Autodesk Fusion 360 part; units mm, degrees
sketch "Sketch1" plane through (0, 0, 0) normal (0, 0, 1) x (1, 0, 0)
  line L0 (0, 0) -> (115, 0)
  line L1 (115, 0) -> (115, 39)
  line L2 (115, 39) -> (0, 39)
  line L3 (0, 39) -> (0, 0)
  circle A0 centre (5, 34) radius 1.6
  circle A1 centre (5, 5) radius 1.6
  circle A2 centre (110, 5) radius 1.6
  circle A3 centre (110, 34) radius 1.6
  dimension "d1" = 115
  dimension "d2" = 39
  dimension "d3" = 3.2
  dimension "d4" = 5
  dimension "d5" = 5
  dimension "d6" = 3.2
  dimension "d7" = 5
  dimension "d8" = 5
  dimension "d9" = 3.2
  dimension "d10" = 3.2
  dimension "d11" = 5
  dimension "d12" = 5
  dimension "d13" = 5
  dimension "d14" = 5
extrude "Extrude1" add sketch "Sketch1" along normal blind 2.7
fillet "Fillet1" radius 6 4 edges at (115, 39, 1.35) (115, 0, 1.35) (0, 39, 1.35) (0, 0, 1.35)
Work out the finished part from the listing and answer in its coordinate system (mm). Give positions to 0.01 mm unless a question says otherwise; leave off trailing zeros. Write each loop counter-clockwise with the first axis right and the second up, starting at its lowest first coordinate (ties: lowest second). Pieces come first, ordered by that corner, then holes.
(1) The part is cut by section B-B on x = 5. Write down the section's boundary in (y, z), plus the area to 3 significant figures.
Final values:
outline: (0.08, 0) - (3.4, 0) - (3.4, 2.7) - (0.08, 2.7) - close; (6.6, 0) - (32.4, 0) - (32.4, 2.7) - (6.6, 2.7) - close; (35.6, 0) - (38.92, 0) - (38.92, 2.7) - (35.6, 2.7) - close
area: 87.6 mm2
(2) A flat-ended cylindrical pin translates along its axis: pin 1 Ø2.5 at (x, y) = (110, 34) entering from -Z. Find the tip coordinate at first contact, or state that the pin passes through.
Final values:
pin 1: passes through
(3) The part is cut by section A-A on y = 34. Write down the section's boundary in (x, z), plus the area to 3 significant figures.
Final values:
outline: (0.08, 0) - (3.4, 0) - (3.4, 2.7) - (0.08, 2.7) - close; (6.6, 0) - (108.4, 0) - (108.4, 2.7) - (6.6, 2.7) - close; (111.6, 0) - (114.92, 0) - (114.92, 2.7) - (111.6, 2.7) - close
area: 293 mm2
(4) The mould has two halves that part along Y. Classify faces 1 (the flat face through (57, 0, 1)), 2 (the flat face through (0, 20, 1)), 3 (the cylindrical face through (108.73, 34.97, 1.33)), 4 (the cylindrical face through (5.86, 3.65, 1.33)): pulls with the +Y half, pulls with the -Y half, needs draft (parallel to the pull), parting line crosses it, or undercut.
Final values:
face 1: pulls with the -Y half
face 2: needs draft
face 3: undercut
face 4: undercut
(5) A straight line is drawn through the part: line 1 (Y direction, x = 110, z = 2.1). Find the intervals that lie inside material, in ascending order.
Final values:
line 1: y = 0.08 to 3.4, 6.6 to 32.4, 35.6 to 38.92
